Could you check a few things on this model? Use its own coordinates, in mm. A direction names the side the tool comes from. Round coordinates to 2 decimals unless told otherwise and drop trailing zeros. Write each loop counter-clockwise with the first axis right and the second up, starting at its lowest first coordinate (ties: lowest second). Pieces come first, ordered by that corner, then holes. Notation, with made-up numbers: (64.5, -34.75) -> (71.5, -34.75) arc R14 cw to (71.5, -10.75) -> close; hole circle Ø6 at (55.25, 64.5). An arc over 180 degrees is marked (long way). Answer in a Markdown table with one row per item. Add a question column.
```python
from build123d import *

# Parameters (mm, degrees)
SKETCH1_W               = 72.11
SKETCH1_H               = 97.4
BOSS_EXTRUDE1_DEPTH     = 2.5
SKETCH2_W               = 5
SKETCH2_H               = 97.4
BOSS_EXTRUDE2_DEPTH     = 6.375
CUT_EXTRUDE1_DEPTH      = 62.240661737
CUT_EXTRUDE1_DEPTH_BACK = 62.240661737
SKETCH3_W               = 40
SKETCH3_H               = 62
CUT_EXTRUDE2_DEPTH      = 77.631155751
CUT_EXTRUDE2_DEPTH_BACK = 77.631155751
SKETCH5_W               = 31.75
SKETCH5_H               = 152.4


with BuildPart() as part:
    # Sketch1 → Boss-Extrude1 (new, symmetric)
    with BuildSketch(Plane(origin=(0, 0, 0), x_dir=(1, 0, 0), z_dir=(0, 1, 0))):
        Rectangle(SKETCH1_W, SKETCH1_H)
    extrude(amount=BOSS_EXTRUDE1_DEPTH, both=True)

    # Sketch2 → Boss-Extrude2 (add, symmetric)
    with BuildSketch(Plane(origin=(0, 0, 0), x_dir=(1, 0, 0), z_dir=(0, 1, 0))):
        with Locations((-33.555, 0)):
            Rectangle(SKETCH2_W, SKETCH2_H)
        with Locations((33.555, 0)):
            Rectangle(SKETCH2_W, SKETCH2_H)
    extrude(amount=BOSS_EXTRUDE2_DEPTH, both=True)

    # Sketch3 → Cut-Extrude1 (cut, two sides: drawn at the far end of the back side and taken through both)
    with BuildSketch(Plane(origin=(0, 2.5, 0), x_dir=(1, 0, 0), z_dir=(0, 1, 0)).offset(-CUT_EXTRUDE1_DEPTH_BACK)):
        Rectangle(SKETCH3_W, SKETCH3_H)
    extrude(amount=CUT_EXTRUDE1_DEPTH + CUT_EXTRUDE1_DEPTH_BACK, mode=Mode.SUBTRACT)

    # Sketch4 → Revolve1 (revolve)
    with BuildSketch(Plane(origin=(0, 0, 0), x_dir=(1, 0, 0), z_dir=(0, 1, 0)), mode=Mode.PRIVATE) as revolve1_sk:
        Polygon((20, 31), (15.058430503, 33.414723774), (30.424854519, 64.86107512), (35.366424016, 62.446351346), align=None)
    revolve1 = revolve(revolve1_sk.sketch.rotate(Axis((20, 0, -31), (0.4390406861851917, 0, -0.8984671813004836)), 180), axis=Axis((20, 0, -31), (0.4390406861851917, 0, -0.8984671813004836)))

    # Mirror1: Revolve1 across plane
    add(revolve1.mirror(Plane.XY))

    # Sketch5 → Cut-Extrude2 (cut, two sides: drawn at the far end of the back side and taken through both)
    with BuildSketch(Plane(origin=(0, 0, 0), x_dir=(1, 0, 0), z_dir=(0, 1, 0)).offset(-CUT_EXTRUDE2_DEPTH_BACK)):
        with Locations((-28.575, 0)):
            Rectangle(SKETCH5_W, SKETCH5_H)
    extrude(amount=CUT_EXTRUDE2_DEPTH + CUT_EXTRUDE2_DEPTH_BACK, mode=Mode.SUBTRACT)


solid = part.part
```
(1) Suppose I cut it at B-B, the plane z = -4.5. Please give me the cut outline in (x, y) (3 decimals).
(2) Suppose I cut it at A-A, the plane x = 7. Please give me the cut outline in (y, z), then the cut area to 3 significant figures.
(3) On a 3-axis mill with a long thin cutter (end or side, diameter ignored), from which of +Z, -Z, +X, -X, +Y, -Y can I reach the whole of each face in a straight line? I mean faces 4 (the face through (20, 4, -31)), 5 (the face through (25, 2.5, -1)), 6 (the face through (3, 0, 31)). Say none if no direction works.
(4) For P1, Ø1, axis at y = 3.5, z = -26, coming from the +X side (3 decimals); P2, Ø1.5, axis at x = 34.5, y = 1.5, coming from the +Z side; P3, Ø1.5, axis at x = -2, y = 0.5, coming from the +Z side, each with a flat end and sliding along its axis, tell me the tip position at first contact or that it passes through.
(5) I need wall thicknesses on L1, parallel to Z at x = 3, y = 0.25; L2, parallel to Y at x = 4, z = 48; L3, parallel to X at y = -1.25, z = 27 (3 decimals). Which ranges of each line are inside material? Lowest first, please.
(6) If we mould it in two halves opening along Z, with no side actions, what happens to faces 1 (the face through (5, 0, 48.7)), 2 (the face through (36.055, 0, 1)), 3 (the face through (-12.7, 0, -40))? For each: pulls with the +Z half, pulls with the -Z half, needs draft (parallel to the pull), parting line crosses it, or undercut.
Response:
| question | item | result |
|---|---|---|
| 1 | outline | (20, -2.5) -> (31.055, -2.5) -> (31.055, -6.375) -> (36.055, -6.375) -> (36.055, 6.375) -> (31.055, 6.375) -> (31.055, 2.5) -> (20, 2.5) -> close |
| 2 | outline | (-2.5, -48.7) -> (2.5, -48.7) -> (2.5, -31) -> (-2.5, -31) -> close; (-2.5, 31) -> (2.5, 31) -> (2.5, 48.7) -> (-2.5, 48.7) -> close |
| 2 | area | 177 mm² |
| 3 | face 4 | -X, +Y |
| 3 | face 5 | +Y |
| 3 | face 6 | -X, +Y, -Y |
| 4 | P1 | x = 36.055 |
| 4 | P2 | z = 63.24 |
| 4 | P3 | z = 48.7 |
| 5 | L1 | -48.7 to -31, 31 to 48.7 |
| 5 | L2 | -2.5 to 2.5 |
| 5 | L3 | 20 to 36.055 |
| 6 | face 1 | pulls with the +Z half |
| 6 | face 2 | undercut |
| 6 | face 3 | needs draft |
